Source: CAD feature listing. Evaluate the final solid. Frame: model axes, mm. Give positions to 0.01 mm unless a question says otherwise; leave off trailing zeros. Loops run counter-clockwise (first coordinate to the right, second up) from the corner with the lowest first, then second, coordinate; pieces in that order, holes last. Notation, with made-up numbers: M 54,33.5 L 95,33.5 A17 cw 95,42.5 Z; hole C 74.25,30.5 d1. An arc over 180 degrees is marked long. Write item = value, one per line.
from build123d import *

# Parameters (mm, degrees)
SKETCH2_R           = 5
BOSS_EXTRUDE1_DEPTH = 10


with BuildPart() as part:
    # Sketch2 → Boss-Extrude1 (new body)
    with BuildSketch(Plane.XY):
        with BuildLine():
            Line((0, 10), (0, -10))
            Line((0, -10), (-15, -10))
            ThreePointArc((-15, -10), (-25, 0), (-15, 10))
            Line((-15, 10), (0, 10))
        make_face()
        with Locations((-15, 0)):
            Circle(SKETCH2_R, mode=Mode.SUBTRACT)
    extrude(amount=-BOSS_EXTRUDE1_DEPTH)


solid = part.part
1. Cut plane D-D, the plane y = -8. Return the cut outline in (x, z), then the cut area to 3 significant figures.
Derived:
outline = M -21,-10 L 0,-10 L 0,0 L -21,0 Z
area = 210 mm²
2. Cut plane A-A, the plane y = 0. Return the cut outline in (x, z), then the cut area to 3 significant figures.
Derived:
outline = M -25,-10 L -20,-10 L -20,0 L -25,0 Z; M -10,-10 L 0,-10 L 0,0 L -10,0 Z
area = 150 mm²
3. Material intervals for probe 1 along Y at (x, z) = (-15, -7); probe 2 along X at (y, z) = (4.5, -5.75); probe 3 along X at (y, z) = (-4, -0.25), sorted ascending. Write a range as from..to.
Derived:
probe_1 = -10..-5, 5..10
probe_2 = -23.93..-17.18, -12.82..0
probe_3 = -24.17..-18, -12..0
4. Pull-direction query (X, two-part tool) for faces 1 (the flat face through (-9.5, 0.1, 0)), 2 (the cylindrical face through (-20, 0, -5)), 3 (the flat face through (0, 0, -5)), 4 (the cylindrical face through (-25, 0, -5)); classes: +X half, -X half, draft (parallel to the pull), parting line (faces both ways), or undercut.
Derived:
face_1 = draft
face_2 = undercut
face_3 = +X half
face_4 = -X half
5. First-contact query: pin 1 Ø4 at (y, z) = (-3, -5.5) entering from -X. Flat tip, straight axial feed; report the tip coordinate or a pass-through.
Derived:
pin_1 = -24.95
6. Cut plane C-C, the plane x = -13. Return the cut outline in (y, z), then the cut area to 3 significant figures.
Derived:
outline = M -10,-10 L -4.58,-10 L -4.58,0 L -10,0 Z; M 4.58,-10 L 10,-10 L 10,0 L 4.58,0 Z
area = 108 mm²
7. Cut plane B-B, the plane z = -7.5. Return the cut outline in (x, y).
Derived:
outline = M -15,-10 L 0,-10 L 0,10 L -15,10 A10 ccw Z; hole C -15,0 d10
